from build123d import *

# Parameters (mm, degrees)
SKETCH_1_R      = 2.5
EXTRUDE_1_DEPTH = 150


with BuildPart() as part:
    # 草图1 → 凸台-拉伸1 (new body)
    with BuildSketch(Plane.XY):
        with BuildLine():
            Line((16.486773435, 27.123343944), (19.340326826, 24.269790554))
            ThreePointArc((19.340326826, 24.269790554), (19.885221932, 24.161404178), (20.193880216, 24.623343944))
            Line((20.193880216, 24.623343944), (20.193880216, 27.043444957))
            Line((20.193880216, 27.043444957), (21.693880216, 27.043444957))
            ThreePointArc((21.693880216, 27.043444957), (22.047433607, 26.896998348), (22.193880216, 26.543444957))
            Line((22.193880216, 26.543444957), (22.193880216, 21.143444957))
            ThreePointArc((22.193880216, 21.143444957), (21.900986997, 20.436338176), (21.193880216, 20.143444957))
            Line((21.193880216, 20.143444957), (15.793880216, 20.143444957))
            ThreePointArc((15.793880216, 20.143444957), (15.440326826, 20.289891566), (15.293880216, 20.643444957))
            Line((15.293880216, 20.643444957), (15.293880216, 22.143444957))
            Line((15.293880216, 22.143444957), (17.713981229, 22.143444957))
            ThreePointArc((17.713981229, 22.143444957), (18.175920995, 22.452103241), (18.06753462, 22.996998348))
            Line((18.06753462, 22.996998348), (15.213981229, 25.850551738))
            ThreePointArc((15.213981229, 25.850551738), (14.88955788, 26.06732449), (14.506874448, 26.143444957))
            Line((14.506874448, 26.143444957), (12.713495459, 26.143444957))
            Line((12.713495459, 26.143444957), (12.193880216, 26.443444957))
            Line((12.193880216, 26.443444957), (11.674264974, 26.143444957))
            Line((11.674264974, 26.143444957), (9.880885985, 26.143444957))
            ThreePointArc((9.880885985, 26.143444957), (9.498202552, 26.06732449), (9.173779204, 25.850551738))
            Line((9.173779204, 25.850551738), (6.320225813, 22.996998348))
            ThreePointArc((6.320225813, 22.996998348), (6.211839437, 22.452103241), (6.673779204, 22.143444957))
            Line((6.673779204, 22.143444957), (9.093880216, 22.143444957))
            Line((9.093880216, 22.143444957), (9.093880216, 20.643444957))
            ThreePointArc((9.093880216, 20.643444957), (8.947433607, 20.289891566), (8.593880216, 20.143444957))
            Line((8.593880216, 20.143444957), (3.193880216, 20.143444957))
            ThreePointArc((3.193880216, 20.143444957), (2.486773435, 20.436338176), (2.193880216, 21.143444957))
            Line((2.193880216, 21.143444957), (2.193880216, 26.543444957))
            ThreePointArc((2.193880216, 26.543444957), (2.340326826, 26.896998348), (2.693880216, 27.043444957))
            Line((2.693880216, 27.043444957), (4.193880216, 27.043444957))
            Line((4.193880216, 27.043444957), (4.193880216, 24.623343944))
            ThreePointArc((4.193880216, 24.623343944), (4.5025385, 24.161404178), (5.047433607, 24.269790554))
            Line((5.047433607, 24.269790554), (7.900986997, 27.123343944))
            ThreePointArc((7.900986997, 27.123343944), (8.117759749, 27.447767293), (8.193880216, 27.830450726))
            Line((8.193880216, 27.830450726), (8.193880216, 29.623829715))
            Line((8.193880216, 29.623829715), (8.493880216, 30.143444957))
            Line((8.493880216, 30.143444957), (8.193880216, 30.663060199))
            Line((8.193880216, 30.663060199), (8.193880216, 32.456439189))
            ThreePointArc((8.193880216, 32.456439189), (8.117759749, 32.839122621), (7.900986997, 33.16354597))
            Line((7.900986997, 33.16354597), (5.047433607, 36.01709936))
            ThreePointArc((5.047433607, 36.01709936), (4.5025385, 36.125485736), (4.193880216, 35.66354597))
            Line((4.193880216, 35.66354597), (4.193880216, 33.243444957))
            Line((4.193880216, 33.243444957), (2.693880216, 33.243444957))
            ThreePointArc((2.693880216, 33.243444957), (2.340326826, 33.389891566), (2.193880216, 33.743444957))
            Line((2.193880216, 33.743444957), (2.193880216, 39.143444957))
            ThreePointArc((2.193880216, 39.143444957), (2.486773435, 39.850551738), (3.193880216, 40.143444957))
            Line((3.193880216, 40.143444957), (8.593880216, 40.143444957))
            ThreePointArc((8.593880216, 40.143444957), (8.947433607, 39.996998348), (9.093880216, 39.643444957))
            Line((9.093880216, 39.643444957), (9.093880216, 38.143444957))
            Line((9.093880216, 38.143444957), (6.673779204, 38.143444957))
            ThreePointArc((6.673779204, 38.143444957), (6.211839437, 37.834786673), (6.320225813, 37.289891566))
            Line((6.320225813, 37.289891566), (9.173779204, 34.436338176))
            ThreePointArc((9.173779204, 34.436338176), (9.498202552, 34.219565425), (9.880885985, 34.143444957))
            Line((9.880885985, 34.143444957), (11.674264974, 34.143444957))
            Line((11.674264974, 34.143444957), (12.193880216, 33.843444957))
            Line((12.193880216, 33.843444957), (12.713495459, 34.143444957))
            Line((12.713495459, 34.143444957), (14.506874448, 34.143444957))
            ThreePointArc((14.506874448, 34.143444957), (14.88955788, 34.219565425), (15.213981229, 34.436338176))
            Line((15.213981229, 34.436338176), (18.06753462, 37.289891566))
            ThreePointArc((18.06753462, 37.289891566), (18.175920995, 37.834786673), (17.713981229, 38.143444957))
            Line((17.713981229, 38.143444957), (15.293880216, 38.143444957))
            Line((15.293880216, 38.143444957), (15.293880216, 39.643444957))
            ThreePointArc((15.293880216, 39.643444957), (15.440326826, 39.996998348), (15.793880216, 40.143444957))
            Line((15.793880216, 40.143444957), (21.193880216, 40.143444957))
            ThreePointArc((21.193880216, 40.143444957), (21.900986997, 39.850551738), (22.193880216, 39.143444957))
            Line((22.193880216, 39.143444957), (22.193880216, 33.743444957))
            ThreePointArc((22.193880216, 33.743444957), (22.047433607, 33.389891566), (21.693880216, 33.243444957))
            Line((21.693880216, 33.243444957), (20.193880216, 33.243444957))
            Line((20.193880216, 33.243444957), (20.193880216, 35.66354597))
            ThreePointArc((20.193880216, 35.66354597), (19.885221932, 36.125485736), (19.340326826, 36.01709936))
            Line((19.340326826, 36.01709936), (16.486773435, 33.16354597))
            ThreePointArc((16.486773435, 33.16354597), (16.270000684, 32.839122621), (16.193880216, 32.456439189))
            Line((16.193880216, 32.456439189), (16.193880216, 30.663060199))
            Line((16.193880216, 30.663060199), (15.893880216, 30.143444957))
            Line((15.893880216, 30.143444957), (16.193880216, 29.623829715))
            Line((16.193880216, 29.623829715), (16.193880216, 27.830450726))
            ThreePointArc((16.193880216, 27.830450726), (16.270000684, 27.447767293), (16.486773435, 27.123343944))
        make_face()
        with Locations((12.193880216, 30.143444957)):
            Circle(SKETCH_1_R, mode=Mode.SUBTRACT)
    extrude(amount=EXTRUDE_1_DEPTH)


solid = part.part
CAD build for the part. Positions are in the model's coordinates, mm. A direction names the side the tool comes from. Round coordinates to 2 decimals unless told otherwise and drop trailing zeros. Write each question's results on one line, items separated by ' | '.
1. Flat gauge pins, fed straight in: P1, Ø8, axis at x = 12.19, y = 30.14, coming from the -Z side; P2, Ø2, axis at x = 11, z = 68, coming from the -Y side; P3, Ø1.4, axis at x = 11, z = 59.5, coming from the +Y side. Where does each tip first touch, or does it go through?
Findings below:
P1: stops at z = 0 | P2: stops at y = 26.14 | P3: stops at y = 34.14
2. Wall check: line 1 along Y through (x, z) = (19, 138); line 2 along X through (y, z) = (38, 137); line 3 along X through (y, z) = (37.5, 61). Give the ranges that are in metal, low to high. Write a range as [from, to].
Findings below:
line 1: y = [20.14, 24.61], [35.68, 40.14] | line 2: x = [2.19, 6.32], [18.06, 22.19] | line 3: x = [2.19, 6.19], [18.19, 22.19]
3. Pull direction Y, two halves, no side cores. Call faces 3 (the face through (20.194, 26, 74)), 4 (the face through (19, 20.143, 74)), 5 (the face through (2.194, 36, 74)): pulls with the +Y half, pulls with the -Y half, needs draft (parallel to the pull), parting line crosses it, or undercut.
Findings below:
face 3: undercut | face 4: pulls with the -Y half | face 5: needs draft
4. 3-axis set-ups, long thin cutter, end or side, ignore diameter. For faces 1 (the face through (4.194, 34, 74)), 2 (the face through (22.194, 36, 74)): which of +Z, -Z, +X, -X, +Y, -Y reach the whole face in a straight line?
Findings below:
face 1: +Z, -Z | face 2: +Z, -Z, +X, +Y, -Y
